```python
from build123d import *
from build123d.topology import SkipClean

# Parameters (mm, degrees)
BOSS_EXTRUDE1_DEPTH = 19.05
SKETCH7_R           = 4.7625
CUT_EXTRUDE7_DEPTH  = 38.1
FILLET4_R           = 38.1
FILLET5_R           = 6.35
SKETCH8_R           = 4.7625
CUT_EXTRUDE8_DEPTH  = 195.283940649
FILLET6_RADIUS      = 9.525
FILLET6_LENGTH      = 19.05
FILLET7_RADIUS      = 9.525
FILLET7_LENGTH      = 19.05
CUT_EXTRUDE9_START  = -19.05
CUT_EXTRUDE9_DEPTH  = 12.7
CUT_EXTRUDE10_START = -19.05
CUT_EXTRUDE10_DEPTH = 12.7
CUT_EXTRUDE11_START = -19.05
CUT_EXTRUDE11_DEPTH = 12.7
SKETCH12_R          = 4.7625
BOSS_EXTRUDE2_DEPTH = 38.1
CUT_EXTRUDE12_DEPTH = 34.925
CUT_EXTRUDE13_START = -6.985
SKETCH13_4_R        = 4.7625
CUT_EXTRUDE13_DEPTH = 24.13
FILLET13_R          = 3.175
FILLET14_R          = 3.175
FILLET15_R          = 3.175


with BuildPart() as part:
    # Sketch1 → Boss-Extrude1 (new body)
    with BuildSketch(Plane(origin=(0, 0, 0), x_dir=(1, 0, 0), z_dir=(0, 1, 0))):
        with BuildLine():
            ThreePointArc((3.175, 0), (0.92993597, -0.92993597), (0, -3.175))
            Line((0, -3.175), (0, -127))
            Line((0, -127), (19.05, -127))
            Line((19.05, -127), (19.05, -111.125))
            ThreePointArc((19.05, -111.125), (19.97993597, -108.87993597), (22.225, -107.95))
            Line((22.225, -107.95), (123.563707018, -107.95))
            ThreePointArc((123.563707018, -107.95), (125.808771048, -108.87993597), (126.738707018, -111.125))
            Line((126.738707018, -111.125), (126.738707018, -127))
            Line((126.738707018, -127), (145.788707018, -127))
            Line((145.788707018, -127), (145.788707018, -87.316702208))
            Line((145.788707018, -87.316702208), (19.05, 0))
            Line((19.05, 0), (3.175, 0))
        make_face()
        with BuildLine():
            Line((29.002606919, -29.990275978), (111.5275446, -86.845877379))
            ThreePointArc((111.5275446, -86.845877379), (113.98824654, -93.961474404), (107.924937681, -98.425))
            Line((107.924937681, -98.425), (25.4, -98.425))
            ThreePointArc((25.4, -98.425), (20.909871939, -96.565128061), (19.05, -92.075))
            Line((19.05, -92.075), (19.05, -35.2193986))
            ThreePointArc((19.05, -35.2193986), (22.446532033, -29.598052945), (29.002606919, -29.990275978))
        make_face(mode=Mode.SUBTRACT)
    extrude(amount=BOSS_EXTRUDE1_DEPTH)

    # Sketch7 → Cut-Extrude7 (cut)
    with BuildSketch(Plane(origin=(0, 0, 0), x_dir=(-1, 0, 0), z_dir=(0, 0, -1))):
        with Locations((-9.525, 9.525)):
            Circle(SKETCH7_R)
    extrude(amount=-CUT_EXTRUDE7_DEPTH, mode=Mode.SUBTRACT)

    # Fillet4
    fillet4_edges = [part.edges().sort_by_distance(p)[0] for p in [
        (145.788707018, 9.525, 87.316702208),
    ]]
    fillet(fillet4_edges, radius=FILLET4_R)

    # Fillet5
    fillet5_edges = [part.edges().sort_by_distance(p)[0] for p in [
        (19.05, 9.525, 0),
    ]]
    fillet(fillet5_edges, radius=FILLET5_R)

    # Sketch8 → Cut-Extrude8 (cut, through all)
    with BuildSketch(Plane.ZY):
        with Locations((117.475, 9.525)):
            Circle(SKETCH8_R)
    extrude(amount=-CUT_EXTRUDE8_DEPTH, mode=Mode.SUBTRACT)

    # Fillet6: full round fillet: the end face becomes a half cylinder, R = half its width
    fillet6_face = Plane((9.525, 9.525, 127), x_dir=(1, 0, 0), z_dir=(0, 0, 1))  # on the end face: x along it, z out of the body
    fillet6_slab = fillet6_face.offset(-FILLET6_RADIUS / 2) * Box(FILLET6_LENGTH, 2 * FILLET6_RADIUS, FILLET6_RADIUS, mode=Mode.PRIVATE)  # the body's end, R deep
    fillet6_round = Plane((9.525, 9.525, 117.475), x_dir=(0, 0, 1), z_dir=(1, 0, 0)) * Cylinder(FILLET6_RADIUS, FILLET6_LENGTH, mode=Mode.PRIVATE)  # its axis R under the face
    add(fillet6_slab - fillet6_round, mode=Mode.SUBTRACT)

    # Fillet7: full round fillet: the end face becomes a half cylinder, R = half its width
    fillet7_face = Plane((136.263707018, 9.525, 127), x_dir=(-1, 0, 0), z_dir=(0, 0, 1))  # on the end face: x along it, z out of the body
    fillet7_slab = fillet7_face.offset(-FILLET7_RADIUS / 2) * Box(FILLET7_LENGTH, 2 * FILLET7_RADIUS, FILLET7_RADIUS, mode=Mode.PRIVATE)  # the body's end, R deep
    fillet7_round = Plane((136.263707018, 9.525, 117.475), x_dir=(0, 0, 1), z_dir=(-1, 0, 0)) * Cylinder(FILLET7_RADIUS, FILLET7_LENGTH, mode=Mode.PRIVATE)  # its axis R under the face
    add(fillet7_slab - fillet7_round, mode=Mode.SUBTRACT)

    # Sketch9 → Cut-Extrude9 (cut)
    with BuildSketch(Plane(origin=(0, 19.05, 0), x_dir=(1, 0, 0), z_dir=(0, 1, 0)).offset(CUT_EXTRUDE9_START)):
        with BuildLine():
            Line((6.985, -44.45), (12.065, -44.45))
            ThreePointArc((12.065, -44.45), (14.31006403, -45.37993597), (15.24, -47.625))
            Line((15.24, -47.625), (15.24, -92.075))
            Line((15.24, -92.075), (15.24, -102.87))
            ThreePointArc((15.24, -102.87), (14.31006403, -105.11506403), (12.065, -106.045))
            Line((12.065, -106.045), (6.985, -106.045))
            ThreePointArc((6.985, -106.045), (4.73993597, -105.11506403), (3.81, -102.87))
            Line((3.81, -102.87), (3.81, -47.625))
            ThreePointArc((3.81, -47.625), (4.73993597, -45.37993597), (6.985, -44.45))
        make_face()
    extrude(amount=CUT_EXTRUDE9_DEPTH, mode=Mode.SUBTRACT)

    # Sketch10 → Cut-Extrude10 (cut)
    with BuildSketch(Plane(origin=(0, 19.05, 0), x_dir=(1, 0, 0), z_dir=(0, 1, 0)).offset(CUT_EXTRUDE10_START)):
        with BuildLine():
            Line((20.6375, -11.763381719), (20.6375, -17.932294237))
            ThreePointArc((20.6375, -17.932294237), (21.001827173, -19.409028221), (22.011196541, -20.546855548))
            Line((22.011196541, -20.546855548), (63.441606739, -49.090359539))
            ThreePointArc((63.441606739, -49.090359539), (65.81797034, -49.598286152), (67.857471509, -48.277101687))
            Line((67.857471509, -48.277101687), (70.739557043, -44.09380359))
            ThreePointArc((70.739557043, -44.09380359), (71.247483656, -41.717439989), (69.926299192, -39.67793882))
            Line((69.926299192, -39.67793882), (25.613803459, -9.148820408))
            ThreePointArc((25.613803459, -9.148820408), (22.335766016, -8.952708891), (20.6375, -11.763381719))
        make_face()
        with BuildLine():
            Line((123.418648971, -80.387093072), (120.536563436, -84.570391169))
            ThreePointArc((120.536563436, -84.570391169), (118.497062267, -85.891575634), (116.120698666, -85.383649021))
            Line((116.120698666, -85.383649021), (71.808202933, -54.854530608))
            ThreePointArc((71.808202933, -54.854530608), (70.487018469, -52.815029439), (70.994945082, -50.438665838))
            Line((70.994945082, -50.438665838), (73.877030616, -46.255367741))
            ThreePointArc((73.877030616, -46.255367741), (75.916531785, -44.934183277), (78.292895386, -45.44210989))
            Line((78.292895386, -45.44210989), (122.605391119, -75.971228302))
            ThreePointArc((122.605391119, -75.971228302), (123.926575583, -78.010729471), (123.418648971, -80.387093072))
        make_face()
    extrude(amount=CUT_EXTRUDE10_DEPTH, mode=Mode.SUBTRACT)

    # Sketch11 → Cut-Extrude11 (cut)
    with BuildSketch(Plane(origin=(0, 19.05, 0), x_dir=(1, 0, 0), z_dir=(0, 1, 0)).offset(CUT_EXTRUDE11_START)):
        with BuildLine():
            Line((117.723743339, -104.14), (138.043743339, -104.14))
            ThreePointArc((138.043743339, -104.14), (140.775902425, -102.582384223), (140.82733452, -99.437831007))
            Line((140.82733452, -99.437831007), (131.819281268, -83.018732847))
            ThreePointArc((131.819281268, -83.018732847), (129.196718657, -81.374987965), (126.421128775, -82.74459838))
            Line((126.421128775, -82.74459838), (115.109182028, -99.163696541))
            ThreePointArc((115.109182028, -99.163696541), (114.913070511, -102.441733984), (117.723743339, -104.14))
        make_face()
    extrude(amount=CUT_EXTRUDE11_DEPTH, mode=Mode.SUBTRACT)

    # Sketch12 → Boss-Extrude2 (add)
    with BuildSketch(Plane.ZY):
        with BuildLine():
            Line((31.761333992, 55.437605021), (31.761333992, 0))
            Line((31.761333992, 0), (81.213525096, 0))
            Line((81.213525096, 0), (81.213525096, 19.05))
            Line((81.213525096, 19.05), (48.843024558, 61.236057633))
            ThreePointArc((48.843024558, 61.236057633), (38.224623085, 64.457114505), (31.761333992, 55.437605021))
        make_face()
        with Locations(Location((41.286333992, 55.437605021, 0), (0, 0, 180))):
            Circle(SKETCH12_R, mode=Mode.SUBTRACT)
    extrude(amount=BOSS_EXTRUDE2_DEPTH)

    # Sketch13 → Cut-Extrude12 (cut)
    with BuildSketch(Plane.ZY.offset(38.1)):
        with BuildLine():
            Line((34.936333992, 39.772832304), (34.936333992, 18.134396169))
            ThreePointArc((34.936333992, 18.134396169), (37.154655789, 15.106956357), (40.709809152, 16.309964245))
            Line((40.709809152, 16.309964245), (57.81580954, 40.673447753))
            ThreePointArc((57.81580954, 40.673447753), (57.910209366, 44.179857475), (54.717843702, 45.633343608))
            Line((54.717843702, 45.633343608), (37.611843313, 42.908296235))
            ThreePointArc((37.611843313, 42.908296235), (35.696120968, 41.833747404), (34.936333992, 39.772832304))
        make_face()
        with BuildLine():
            Line((41.668763699, 3.175), (73.114694638, 3.175))
            ThreePointArc((73.114694638, 3.175), (75.78099304, 4.626202497), (76.009912608, 7.653202941))
            Line((76.009912608, 7.653202941), (64.11901518, 34.070224292))
            ThreePointArc((64.11901518, 34.070224292), (61.563303547, 35.923817266), (58.671896573, 34.656049709))
            Line((58.671896573, 34.656049709), (39.116863062, 8.239028358))
            ThreePointArc((39.116863062, 8.239028358), (38.833425091, 4.921196311), (41.668763699, 3.175))
        make_face()
    extrude(amount=-CUT_EXTRUDE12_DEPTH, mode=Mode.SUBTRACT)

    # Sketch13<4> → Cut-Extrude13 (cut)
    # profile 1 of 3: a face of its own
    with SkipClean():  # the faces are left unmerged after this step: merging them gives an invalid solid
        with BuildSketch(Plane.ZY.offset(38.1).offset(CUT_EXTRUDE13_START)):
            with BuildLine():
                Line((37.611843313, 42.908296235), (54.717843702, 45.633343608))
                ThreePointArc((54.717843702, 45.633343608), (57.910209366, 44.179857475), (57.81580954, 40.673447753))
                Line((57.81580954, 40.673447753), (40.709809152, 16.309964245))
                ThreePointArc((40.709809152, 16.309964245), (37.154655789, 15.106956357), (34.936333992, 18.134396169))
                Line((34.936333992, 18.134396169), (34.936333992, 39.772832304))
                ThreePointArc((34.936333992, 39.772832304), (35.696120968, 41.833747404), (37.611843313, 42.908296235))
            make_face()
        # profile 2 of 3: a face of its own
        with BuildSketch(Plane.ZY.offset(38.1).offset(CUT_EXTRUDE13_START)):
            with BuildLine():
                Line((31.761333992, 44.275117198), (58.579423638, 48.547335312))
                Line((58.579423638, 48.547335312), (48.843044303, 61.236059961))
                ThreePointArc((48.843044303, 61.236059961), (38.22461551, 64.457129972), (31.761316911, 55.437590446))
                Line((31.761316911, 55.437590446), (31.761333992, 44.275117198))
            make_face()
            with Locations(Location((41.286333992, 55.437605021, 0), (0, 0, 180))):
                Circle(SKETCH13_4_R, mode=Mode.SUBTRACT)
        # profile 3 of 3: a face of its own
        with BuildSketch(Plane.ZY.offset(38.1).offset(CUT_EXTRUDE13_START)):
            with BuildLine():
                Line((39.116863062, 8.239028358), (58.671896573, 34.656049709))
                ThreePointArc((58.671896573, 34.656049709), (61.563303547, 35.923817266), (64.11901518, 34.070224292))
                Line((64.11901518, 34.070224292), (76.009912608, 7.653202941))
                ThreePointArc((76.009912608, 7.653202941), (75.78099304, 4.626202497), (73.114694638, 3.175))
                Line((73.114694638, 3.175), (41.668763699, 3.175))
                ThreePointArc((41.668763699, 3.175), (38.833425091, 4.921196311), (39.116863062, 8.239028358))
            make_face()
        extrude(amount=-CUT_EXTRUDE13_DEPTH, mode=Mode.SUBTRACT)
    add(part.part.scale(1), mode=Mode.REPLACE)  # the faces are merged on a copy

    # Fillet13
    fillet13_edges = [part.edges().sort_by_distance(p)[0] for p in [
        (-19.05, 44.275117198, 31.761333992),
        (-19.05, 48.547335312, 58.579423638),
    ]]
    fillet(fillet13_edges, radius=FILLET13_R)

    # Fillet14
    fillet14_edges = [part.edges().sort_by_distance(p)[0] for p in [
        (-19.05, 0, 31.761333992),
    ]]
    fillet(fillet14_edges, radius=FILLET14_R)

    # Fillet15
    # the kernel refuses this fillet: 3.175 mm, written as the material it takes off along each edge
    with BuildSketch(Plane(origin=(0, 19.05, 81.213525096), x_dir=(0, 0.7933533402912315, -0.6087614290087253), z_dir=(-1, 0, 0))) as fillet15_piece_1:
        with BuildLine():
            CenterArc((FILLET15_R * 0.339454258863, FILLET15_R), FILLET15_R, 232.5, 37.5)
            Line((-FILLET15_R * 0.269307170145, FILLET15_R * 0.206646659709), (0, 0))
            Line((0, 0), (FILLET15_R * 0.339454258863, 0))
        make_face()
    extrude(amount=40.79441818, mode=Mode.SUBTRACT)
    with BuildSketch(Plane(origin=(0, 0, 81.213525096), x_dir=(0, 0, -1), z_dir=(-1, 0, 0))) as fillet15_piece_2:
        with BuildLine():
            CenterArc((FILLET15_R, -FILLET15_R), FILLET15_R, 90, 90)
            Line((0, -FILLET15_R), (0, 0))
            Line((0, 0), (FILLET15_R, 0))
        make_face()
    extrude(amount=46.0375, mode=Mode.SUBTRACT)


solid = part.part
```
For this review, take the finished solid that the model builds, in its own axes (mm). A direction names the side the tool comes from. Round coordinates to 2 decimals unless told otherwise and drop trailing zeros. Order: outer loops, then holes, each group sorted by start corner. A loop starts at its lowest first (then second) coordinate and runs counter-clockwise, first axis right, second up.
Q1. We need section C-C, the plane y = 26.5. Give the boundary of the cut face in (x, z) (3 decimals).
Findings below:
outline: (-38.1, 31.761) - (0, 31.761) - (0, 75.497) - (-38.1, 75.497) - (-38.1, 67.527) - (-3.175, 67.527) - (-3.175, 52.634) - (-38.1, 52.634) - (-38.1, 47.864) - (-3.175, 47.864) - (-3.175, 34.936) - (-38.1, 34.936) - close
Q2. Mouldability with a two-part tool opening along X and no side actions: class faces 4 (the cylindrical face through (-20.882, 15.124, 37.101)), 5 (the cylindrical face through (10.557, 4.876, 18.783)), 6 (the flat face through (-3.175, 34, 44)) as pulls with the +X half, pulls with the -X half, needs draft (parallel to the pull), parting line crosses it, or undercut.
Findings below:
face 4: needs draft
face 5: undercut
face 6: pulls with the -X half
Q3. Wall thickness on line 1 (Z direction, x = 118.5, y = 9.5); line 2 (Y direction, x = -5, z = 45) (3 decimals); line 3 (Z direction, x = -26.5, y = 32.5): over which ranges is each line inside the solid? List them lowest first.
Findings below:
line 1: z = 68.52 to 73.14, 85.89 to 94.24, 104.14 to 107.95
line 2: y = 0 to 3.175, 16.187 to 22.42, 44.085 to 52.456, 58.419 to 64.209
line 3: z = 31.76 to 34.94, 52.08 to 57.08, 64.83 to 70.89
Q4. Insertion check: P1, Ø4, axis at x = 131.5, y = 7, coming from the -Z side; P2, Ø5, axis at y = 7.5, z = 15.5, coming from the +X side; P3, Ø1, axis at x = -19.5, z = 72.5, coming from the +Y side. Each pin has a flat end and moves straight along its axis. Give the tip position at first contact, or say it passes through.
Findings below:
P1: stops at z = 76.1
P2: stops at x = 45.18
P3: stops at y = 31.06
Q5. We need section A-A, the plane x = 58. Give the boundary of the cut face in (y, z) (3 decimals), plus the area to 3 significant figures.
Findings below:
outline: (0, 26.835) - (19.05, 26.835) - (19.05, 49.968) - (0, 49.968) - (0, 45.341) - (12.7, 45.341) - (12.7, 31.461) - (0, 31.461) - close; (0, 98.425) - (19.05, 98.425) - (19.05, 107.95) - (0, 107.95) - close
area: 446 mm2
Q6. Machinability: for faces 1 (the flat face through (100.139, 6.261, 60.493)), 2 (the flat face through (-20.88, 44.29, 46.28)), 3 (the flat face through (-19.22, 46.45, 45.42)), which of the approach directions +Z, -Z, +X, -X, +Y, -Y give a long, thin tool a straight path to every point of the face, cutting with its end or side? Answer none if there is none.
Findings below:
face 1: -Y
face 2: -X
face 3: -Z, +Y
